Verification items for the finished model (mm, model axes). A direction names the side the tool comes from. Round coordinates to 2 decimals unless told otherwise and drop trailing zeros. Loops run counter-clockwise (first coordinate to the right, second up) from the corner with the lowest first, then second, coordinate; pieces in that order, holes last. Notation, with made-up numbers: M 30.25,5.5 L 69.25,5.5 A26 cw 69.25,33.5 Z; hole C -18.75,34.25 d2. An arc over 180 degrees is marked long. One line per item, written item: value.
Autodesk Inventor part; units mm, degrees
ref_plane "YZ Plane" through (0, 0, 0) normal (1, 0, 0) x (0, 1, 0)
ref_plane "XZ Plane" through (0, 0, 0) normal (0, 1, 0) x (-1, 0, 0)
ref_plane "XY Plane" through (0, 0, 0) normal (0, 0, 1) x (1, 0, 0)
sketch "Sketch1" plane through (0, 0, 0) normal (1, 0, 0) x (0, 1, 0)
  circle A0 centre (0, 0) radius 32.5
  dimension "d1" = 65
extrude "Extrusion3" add sketch "Sketch1" along normal blind 5
sketch "Sketch3" plane through (5, 0, 0) normal (1, 0, 0) x (0, 0, -1)
  circle A0 centre (0, 0) radius 25
  dimension "d9" = 50
extrude "Extrusion4" add sketch "Sketch3" along normal blind 20
sketch "Sketch4" plane through (25, 0, 0) normal (1, 0, 0) x (0, 0, -1)
  circle A0 centre (0, 0) radius 25
  circle A1 centre (0, 0) radius 32.5
  dimension "d12" = 65
extrude "Extrusion5" add sketch "Sketch4" along normal blind 5 contours A0 | A1
sketch "Sketch5" plane through (0, 0, 0) normal (-1, 0, 0) x (0, 0, 1)
  point P0 (0, 0)
equation "\"d12\" = d1"
properties part number "pully"
(1) Tool access check on faces 4 (the face through (14.86, -7.509, -23.846)), 5 (the face through (2.46, 31, -9.76)). Record the directions out of +Z, -Z, +X, -X, +Y, -Y that give a thin tool (end or side, any length) a straight path to the whole face; none if there is none.
Completed:
face 4: none
face 5: +X, -X
(2) Mould release check, pull along X, two halves, no side actions. Record for faces 1 (the face through (0, 0, 0)), 2 (the face through (30, 0, 0)), 3 (the face through (25, -19, -17)): +X half, -X half, draft (parallel to the pull), parting line (faces both ways), or undercut.
Completed:
face 1: -X half
face 2: +X half
face 3: undercut
(3) Depth check by flat-ended pin: pin 1 Ø12 at (x, z) = (13, -0.5) entering from +Y; pin 2 Ø1.5 at (x, y) = (12.5, 6.5) entering from -Z; pin 3 Ø5 at (x, z) = (3, 21) entering from -Y. Enter the tip coordinate at first touch or a pass-through.
Completed:
pin 1: stops at y = 25
pin 2: stops at z = -24.33
pin 3: stops at y = -26.72
(4) Sectioned sample at C-C on z = 27. Enter the section's corners in (x, y).
Completed:
outline: M 0,-18.09 L 5,-18.09 L 5,18.09 L 0,18.09 Z; M 25,-18.09 L 30,-18.09 L 30,18.09 L 25,18.09 Z
(5) Sectioned sample at D-D on x = 15. Enter the section's corners in (y, z), and give its area (3 significant figures).
Completed:
outline: C 0,0 d50
area: 1,960 mm^2
(6) Thickness scan on L1, parallel to X at y = -17.5, z = 19.5; L2, parallel to Z at x = 3, y = 1; L3, parallel to Z at x = 10, y = 13.5. Record the ranges inside material, lowest first. Write a range as from..to.
Completed:
L1: x = 0..5, 25..30
L2: z = -32.48..32.48
L3: z = -21.04..21.04
(7) Sectioned sample at A-A on z = 0. Enter the section's corners in (x, y).
Completed:
outline: M 0,-32.5 L 5,-32.5 L 5,-25 L 25,-25 L 25,-32.5 L 30,-32.5 L 30,32.5 L 25,32.5 L 25,25 L 5,25 L 5,32.5 L 0,32.5 Z
